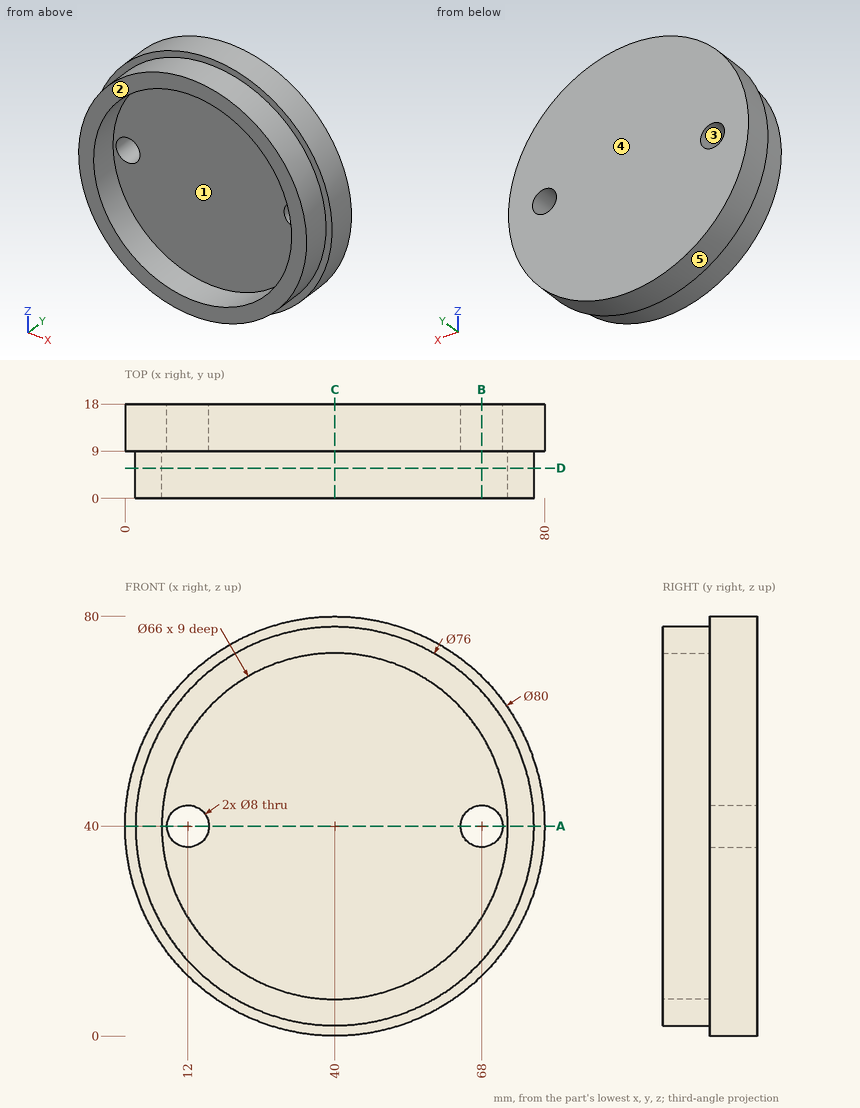
Here's the drawing with two shaded views (mm, measured from the low corner). I have some questions. A direction names the side the tool comes from. Give positions to 0.01 mm unless a question says otherwise; leave off trailing zeros. Order: outer loops, then holes, each group sorted by start corner. A loop starts at its lowest first (then second) coordinate and runs counter-clockwise, first axis right, second up. Notation, with made-up numbers: (25.25, 80.5) - (62.25, 80.5) arc R21 cw to (62.25, 93.5) - close; hole circle Ø10 at (-17, -36.75). An arc over 180 degrees is marked (long way). Use a Markdown table: item, result. Add a question column.
Q1. If we section it at A-A on z = 40: Write out the boundary of the cut face in (x, y).
Q2. If we section it at B-B on x = 68: Write out the boundary of the cut face in (y, z), plus the area to 3 significant figures.
Q3. Please list where these lines run through material, in increasing order: line 1 along X through (y, z) = (12.5, 40); line 2 along X through (y, z) = (2.5, 40); line 3 along Y through (x, z) = (20, 53.5).
Q4. If we section it at D-D on y = 5.75: Write out the boundary of the cut face in (x, z), plus the area to 3 significant figures.
Q5. If we mould it in two halves opening along X, with no side actions, what happens to the marked faces 3, 4 and 5? For each: released by +X, released by -X, zero draft, split by the parting line, or undercut.
Q6. On a 3-axis mill with a long thin cutter (end or side, diameter ignored), from which of +Z, -Z, +X, -X, +Y, -Y can I reach the whole of each face in a straight line? I mean the marked faces 1 and 2. Say none if no direction works.
Q7. If we section it at C-C on x = 40: Write out the boundary of the cut face in (y, z), plus the area to 3 significant figures.
Q8. I'm going to push flat-ended pins straight in: pin 1 (1.5 mm diameter, centred on y = 14.5, z = 34.5, fed in from +X); pin 2 (2 mm diameter, centred on x = 24.5, z = 37, fed in from -Y); pin 3 (6.5 mm diameter, centred on x = 68, z = 40, fed in from +Y); pin 4 (4 mm diameter, centred on x = 59.5, y = 11.5, fed in from +Z). Where does each tip first touch, or does it pass through?
Answers follow:
| question | item | result |
|---|---|---|
| 1 | outline | (0, 9) - (2, 9) - (2, 0) - (7, 0) - (7, 9) - (8, 9) - (8, 18) - (0, 18) - close; (16, 9) - (64, 9) - (64, 18) - (16, 18) - close; (72, 9) - (73, 9) - (73, 0) - (78, 0) - (78, 9) - (80, 9) - (80, 18) - (72, 18) - close |
| 2 | outline | (0, 14.31) - (9, 14.31) - (9, 11.43) - (18, 11.43) - (18, 36) - (9, 36) - (9, 22.54) - (0, 22.54) - close; (0, 57.46) - (9, 57.46) - (9, 44) - (18, 44) - (18, 68.57) - (9, 68.57) - (9, 65.69) - (0, 65.69) - close |
| 2 | area | 590 mm^2 |
| 3 | line 1 | x = 0 to 8, 16 to 64, 72 to 80 |
| 3 | line 2 | x = 2 to 7, 73 to 78 |
| 3 | line 3 | y = 9 to 18 |
| 4 | outline | circle Ø76 at (40, 40); hole circle Ø66 at (40, 40) |
| 4 | area | 1,120 mm^2 |
| 5 | face 3 | undercut |
| 5 | face 4 | zero draft |
| 5 | face 5 | split by the parting line |
| 6 | face 1 | -Y |
| 6 | face 2 | +Z, -Z, +X, -X, -Y |
| 7 | outline | (0, 2) - (9, 2) - (9, 0) - (18, 0) - (18, 80) - (9, 80) - (9, 78) - (0, 78) - (0, 73) - (9, 73) - (9, 7) - (0, 7) - close |
| 7 | area | 810 mm^2 |
| 8 | pin 1 | stops at x = 79.72 |
| 8 | pin 2 | stops at y = 9 |
| 8 | pin 3 | passes through |
| 8 | pin 4 | stops at z = 75.97 |
